Autodesk Inventor part; units mm, degrees
ref_plane "YZ Plane" through (0, 0, 0) normal (1, 0, 0) x (0, 1, 0)
ref_plane "XZ Plane" through (0, 0, 0) normal (0, 1, 0) x (-1, 0, 0)
ref_plane "XY Plane" through (0, 0, 0) normal (0, 0, 1) x (1, 0, 0)
sketch "Sketch6" plane through (0, 0, 0) normal (1, 0, 0) x (0, 1, 0)
  circle A0 centre (0, 0) radius 9.5
  circle A1 centre (-15, -39.2301) radius 16
  circle A2 centre (-15, 39.2301) radius 16
  line L0 (0, 0) -> (0, -14.5947) construction
  line L1 (0, 0) -> (0, -33.02)
  line L2 (0, 0) -> (33.02, 0) construction
  circle A3 centre (0, -33.02) radius 30
  line L3 (0, 0) -> (0, 33.02)
  line L4 (0, 0) -> (33.02, 0) construction
  circle A4 centre (0, 33.02) radius 30
  line L5 (0, 0) -> (-15, -39.2301)
  line L6 (0, 0) -> (-15, 39.2301)
  circle A5 centre (-15, 39.2301) radius 27.5
  circle A6 centre (-15, -39.2301) radius 27.5
  line L7 (30, 33.02) -> (30, -33.02)
  line L8 (-42.5, 39.2301) -> (-42.5, -39.2301)
  line L9 (-8.5189, 65.9555) -> (7.0703, 62.1749)
  line L10 (-8.5189, -65.9555) -> (7.0703, -62.1749)
  dimension "d45" = 19
  dimension "d46" = 32
  dimension "d47" = 32
  dimension "d50" = 15
  dimension "d51" = 15
  dimension "d52" = 33.02
  dimension "d53" = 90
  dimension "d54" = 60
  dimension "d55" = 33.02
  dimension "d56" = 90
  dimension "d57" = 60
  dimension "d58" = 42
  dimension "d59" = 42
  dimension "d60" = 55
  dimension "d61" = 55
extrude "Extrusion6" add sketch "Sketch6" along normal blind 7
sketch "Sketch7" plane through (7, 0, 0) normal (1, 0, 0) x (0, 0, -1)
  circle A0 centre (0, 0) radius 9.5
  circle A1 centre (39.2301, -15) radius 16
  circle A2 centre (-39.2301, -15) radius 16
  line L0 (0, 0) -> (39.2301, -15) construction
  line L1 (0, 0) -> (-39.2301, -15) construction
  dimension "d64" = 19
  dimension "d65" = 32
  dimension "d66" = 32
  dimension "d67" = 15
  dimension "d69" = 15
  dimension "d70" = 42
  dimension "d71" = 42
extrude "Extrusion7" cut sketch "Sketch7" against normal blind 10
sketch "Sketch8" plane through (7, 0, 0) normal (1, 0, 0) x (0, 0, -1)
  circle A0 centre (-66.02, 20) radius 4.25
  circle A1 centre (66.02, 20) radius 4.25
  circle A2 centre (0, -35) radius 4.25
  circle A3 centre (-66.02, 20) radius 10
  circle A4 centre (66.02, 20) radius 10
  circle A5 centre (0, -35) radius 8
  point P0 (0, 0)
  dimension "d74" = 20
  dimension "d75" = 20
  dimension "d76" = 16
extrude "Extrusion8" add sketch "Sketch8" against normal blind 7 contours A3 | A4
fillet "Fillet3" radius 20 4 edges at (3.5, 19.2254, 56.05) (3.5, 11.52, 60.72) (3.5, 19.2254, -56.05) (3.5, 11.52, -60.72)
sketch "Sketch9" plane through (7, 0, 0) normal (1, 0, 0) x (0, 0, -1)
  circle A0 centre (0, -35) radius 4.25
  point P0 (0, 0)
extrude "Extrusion9" cut sketch "Sketch9" against normal blind 10
properties part number "Gearbox Plate 1" material "Aluminum 6061"
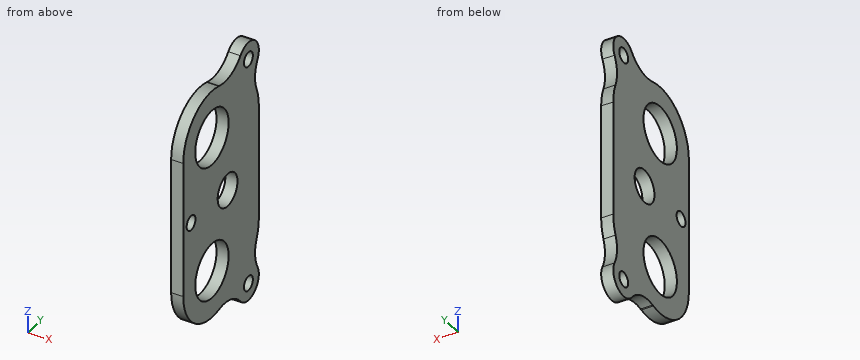
Part model, mm, in its own coordinate system. Coordinates: 2 decimals unless noted, no trailing zeros. Order: outer loops, then holes, each group sorted by start corner. A loop starts at its lowest first (then second) coordinate and runs counter-clockwise, first axis right, second up. Notation, with made-up numbers: (43.25, -13.75) - (53.25, -13.75) arc R27 cw to (53.25, 25.25) - close; hole circle Ø3 at (52, 42.25). An arc over 180 degrees is marked (long way). Use CSV: the item, a comma, the result in double quotes.
Item 1: Saw through at C-C on z = -36.5. Give the cut face in (x, y), and give its area (3 significant figures).
Solved:
outline,"(0, -42.5) - (7, -42.5) - (7, -30.77) - (0, -30.77) - close; (0, 0.77) - (7, 0.77) - (7, 29.8) - (0, 29.8) - close"
area,"285 mm²"
Item 2: Probe probe 1 along Y at (x, z) = (3.75, 0); probe 2 along Z at (x, y) = (2, 19.5); probe 3 along Z at (x, y) = (2, -5). List the from-to ranges inside material, lowest first.
Solved:
probe 1,"y = -42.5 to -39.25, -30.75 to -9.5, 9.5 to 30"
probe 2,"z = -76.01 to -70.24, -61.8 to 61.8, 70.24 to 76.01"
probe 3,"z = -65.31 to -51.72, -26.74 to -8.08, 8.08 to 26.74, 51.72 to 65.31"
Item 3: Drop flat-ended pins along their axis: P1, Ø17, axis at y = 0, z = 0, coming from the -X side; P2, Ø3, axis at x = 3, y = 6, coming from the +Z side; P3, Ø3, axis at x = 2, z = -47.5, coming from the -Y side; P4, Ø2, axis at x = 2, y = -18.5, coming from the +Z side. Give the stop position or say it passes through.
Solved:
P1,"passes through"
P2,"stops at z = 68.23"
P3,"stops at y = -41.65"
P4,"stops at z = 66.62"
Item 4: Saw through at D-D on y = -3. Give the number of separate pieces and of enclosed holes in the cut face, and give its area (3 significant figures).
Solved:
separate pieces,"4"
enclosed holes,"0"
area,"490 mm²"
Item 5: Saw through at B-B on y = -32.5. Give the cut face in (x, z).
Solved:
outline,"(0, -60.44) - (7, -60.44) - (7, -3.44) - (0, -3.44) - close; (0, 3.44) - (7, 3.44) - (7, 60.44) - (0, 60.44) - close"
Item 6: Saw through at A-A on z = 0. Give the cut face in (x, y).
Solved:
outline,"(0, -42.5) - (7, -42.5) - (7, -39.25) - (0, -39.25) - close; (0, -30.75) - (7, -30.75) - (7, -9.5) - (0, -9.5) - close; (0, 9.5) - (7, 9.5) - (7, 30) - (0, 30) - close"
